```python
from build123d import *

# Parameters (mm, degrees)
F1_DEPTH = 749.3
F3_DEPTH = 31.751
F5_DEPTH = 50.8


with BuildPart() as f1:
    # F0 (on Front) → F1 (new body)
    with BuildSketch(Plane.XZ):
        with BuildLine():
            Line((0, -25.4), (0, 0))
            Line((0, 0), (25.4, 0))
            ThreePointArc((25.4, 0), (23.5401280605, 4.4901280605), (19.05, 6.35))
            Line((19.05, 6.35), (0, 6.35))
            ThreePointArc((0, 6.35), (-4.4901280605, 4.4901280605), (-6.35, 0))
            Line((-6.35, 0), (-6.35, -19.05))
            ThreePointArc((-6.35, -19.05), (-4.4901280605, -23.5401280605), (0, -25.4))
        make_face()
    extrude(amount=F1_DEPTH)

    # F2 (on face) → F3 (cut, through all)
    with BuildSketch(Plane(origin=(-6.35, 0, 0), x_dir=(0, -1, 0), z_dir=(-1, 0, 0))):
        Polygon((749.3, -25.4), (749.3, 6.35), (717.55, -25.4), align=None)
    extrude(amount=-F3_DEPTH, mode=Mode.SUBTRACT)

    # F4 (on face) → F5 (cut)
    with BuildSketch(Plane(origin=(-6.35, 0, 0), x_dir=(0, -1, 0), z_dir=(-1, 0, 0))):
        Polygon((31.75, -25.4), (25.4, -19.05), (0, -19.05), (0, -25.4), align=None)
        Polygon((25.4, -19.05), (6.35, 0), (0, 0), (0, -19.05), align=None)
        Polygon((6.35, 0), (0, 6.35), (0, 0), align=None)
    extrude(amount=-F5_DEPTH, mode=Mode.SUBTRACT)


solid = f1.part
```
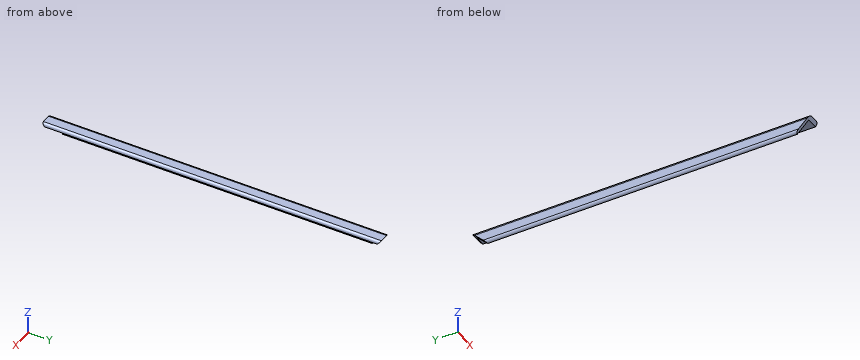
CAD build for the part. Positions are in the model's coordinates, mm. Give positions to 0.01 mm unless a question says otherwise; leave off trailing zeros. Loops run counter-clockwise (first coordinate to the right, second up) from the corner with the lowest first, then second, coordinate; pieces in that order, holes last. Notation, with made-up numbers: (83.25, 58.25) -> (115.25, 58.25) arc R21 ccw to (115.25, 68.25) -> close; hole circle Ø5 at (75.25, 14.25). An arc over 180 degrees is marked (long way). Use a Markdown table: item, result.
1. Wall check: L1, parallel to X at y = -479.5, z = -19; L2, parallel to Z at x = 2.5, y = -349.5; L3, parallel to X at y = -145, z = -19.5. Give the ranges that are in metal, low to high. Write a range as [from, to].
Check result:
| item | result |
|---|---|
| L1 | x = [-6.35, 0] |
| L2 | z = [0, 6.35] |
| L3 | x = [-6.33, 0] |
2. Slice it at C-C (x = 6.5). List the corners of the cut face in (y, z), plus the area to 3 significant figures.
Check result:
| item | result |
|---|---|
| outline | (-749.3, 6.35) -> (-742.95, 0) -> (-6.35, 0) -> (0, 6.35) -> close |
| area | 4,720 mm^2 |
3. Flat gauge pins, fed straight in: pin 1 (1.5 mm diameter, centred on y = -618.5, z = -19.5, fed in from +X); pin 2 (4 mm diameter, centred on x = -0.5, z = -1, fed in from +Y); pin 3 (4 mm diameter, centred on x = 2.5, y = -212.5, fed in from -Z). Where does each tip first touch, or does it go through?
Check result:
| item | result |
|---|---|
| pin 1 | stops at x = 0 |
| pin 2 | stops at y = -5.35 |
| pin 3 | stops at z = 0 |
4. Slice it at A-A (y = -93). List the corners of the cut face in (x, z).
Check result:
| item | result |
|---|---|
| outline | (-6.35, -19.05) arc R6.35 ccw to (0, -25.4) -> (0, 0) -> (25.4, 0) arc R6.35 ccw to (19.05, 6.35) -> (0, 6.35) arc R6.35 ccw to (-6.35, 0) -> close |
5. Slice it at B-B (z = -8). List the corners of the cut face in (x, y), plus the area to 3 significant figures.
Check result:
| item | result |
|---|---|
| outline | (-6.35, -734.95) -> (0, -734.95) -> (0, -14.35) -> (-6.35, -14.35) -> close |
| area | 4,580 mm^2 |
